Answer from the drawing. Dimensions are ordinates in mm from the lowest x, y and z of the part. A direction names the side the tool comes from. Coordinates: 2 decimals unless noted, no trailing zeros. Write each loop counter-clockwise with the first axis right and the second up, starting at its lowest first coordinate (ties: lowest second). Pieces come first, ordered by that corner, then holes. Notation, with made-up numbers: (-10.5, 3) - (7.5, 3) arc R16 cw to (7.5, 14) - close; hole circle Ø1 at (85.25, 39). An arc over 180 degrees is marked (long way). Return JSON: item names as keys, results as strings.
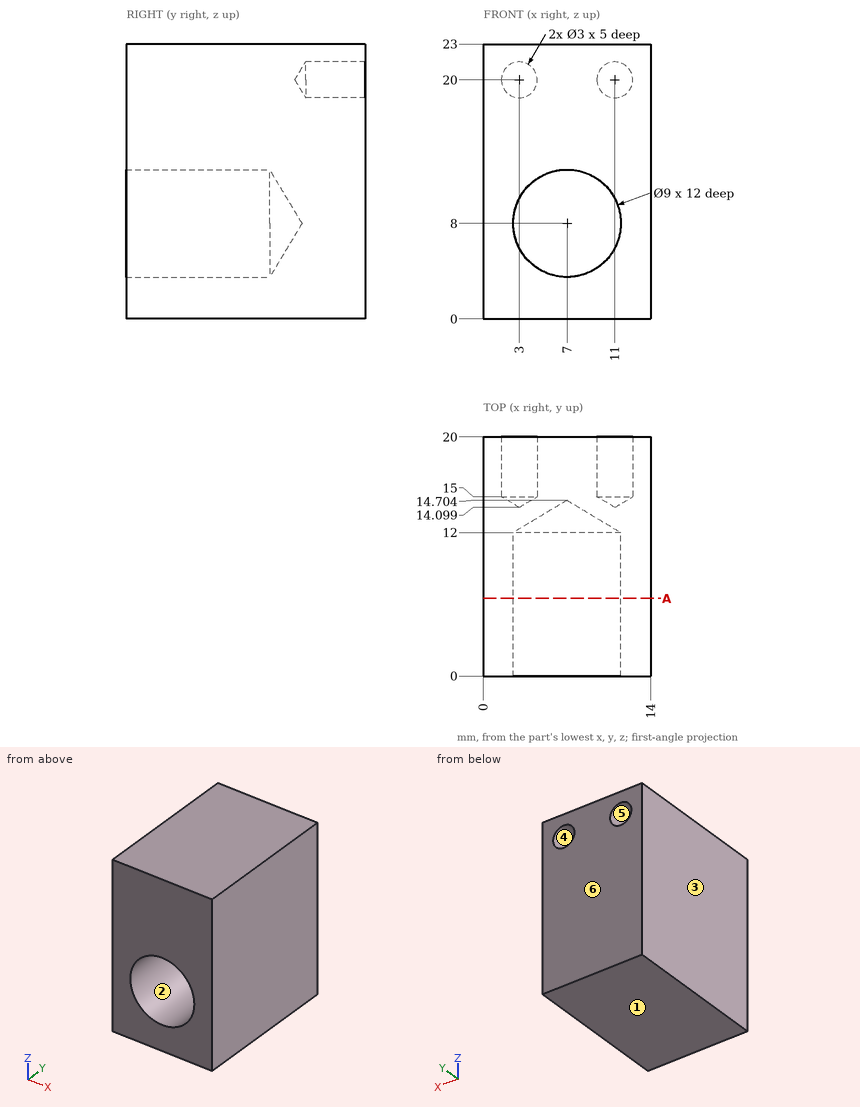
(1) Which of the six approach directions +Z, -Z, +X, -X, +Y, -Y give full straight-line access (tool end or side, diameter ignored) to the marked faces 5 and 6?
Answer:
{"face 5": "+Y", "face 6": "+Z, -Z, +X, -X, +Y"}
(2) Determine the mould class of the marked faces 1, 2, 3 and 4 for opening direction X: +X half, -X half, draft (parallel to the pull), parting line (faces both ways), or undercut.
Answer:
{"face 1": "draft", "face 2": "undercut", "face 3": "-X half", "face 4": "undercut"}
(3) Straight lines are drawn through the part: line 1 (X direction, y = 18.3, z = 20); line 2 (Z direction, x = 7, y = 4.25); line 3 (Z direction, x = 3, y = 18.3). For each, find the intervals that lie inside material, in ascending order. Write a range as from..to.
Answer:
{"line 1": "0..1.5, 4.5..9.5, 12.5..14", "line 2": "0..3.5, 12.5..23", "line 3": "0..18.5, 21.5..23"}
(4) A cutting plane is placed at A-A (y = 6.5). Determine the outline of the cut face in (x, z).
Answer:
{"outline": "(0, 0) - (14, 0) - (14, 23) - (0, 23) - close; hole circle Ø9 at (7, 8)"}
